Check sheet for the modelled part. Datum: model origin and axes. Units: mm. A direction names the side the tool comes from. Coordinates: 2 decimals unless noted, no trailing zeros. Loops run counter-clockwise (first coordinate to the right, second up) from the corner with the lowest first, then second, coordinate; pieces in that order, holes last. Notation, with made-up numbers: (87.5, 53) - (144.5, 53) arc R5 cw to (144.5, 58) - close; hole circle Ø5 at (38.5, -37). An arc over 180 degrees is marked (long way). Use a Markdown table: item, result. Add a question column.
1) Thickness scan on line 1 (Y direction, x = 12, z = 7.2); line 2 (X direction, y = -1.75, z = 7.5); line 3 (Z direction, x = 10.5, y = 7.25). Record the ranges inside material, lowest first.
2) Sectioned sample at B-B, the plane z = 3.75. Enter the section's corners in (x, y), then the cut area to 3 significant figures.
3) Sectioned sample at A-A, the plane z = -0.75. Enter the section's corners in (x, y).
4) Draft check along Y on faces 5 (the flat face through (12, 4, 5)), 6 (the flat face through (-12, 0, 4)), 7 (the cylindrical face through (9.5, -3.9, 7)), 8 (the flat face through (0, -8, 3)). Enter one of: pulls with the +Y half, pulls with the -Y half, needs draft (parallel to the pull), parting line crosses it, or undercut.
5) Sectioned sample at D-D, the plane y = 4. Enter the section's corners in (x, z).
6) Sectioned sample at C-C, the plane x = -12. Enter the section's corners in (y, z).
7) Go/stop test with flat-tipped pins: P1, Ø2, axis at y = 0.5, z = 7.5, coming from the -X side; P2, Ø4, axis at x = 12, y = -4, coming from the -Z side; P3, Ø4, axis at x = -10.5, y = -4.5, coming from the +Z side. Record where each tip stops, or that it passes through.
8) Tool access check on faces 1 (the flat face through (12, -4, 0)), 2 (the cylindrical face through (-1.615, 4.751, 10.986)), 3 (the flat face through (8, 2, 7)), 4 (the flat face through (-8, -4, -2)). Record the directions out of +Z, -Z, +X, -X, +Y, -Y that give a thin tool (end or side, any length) a straight path to the whole face; none if there is none.
from build123d import *

# Parameters (mm, degrees)
F0_W     = 8
F0_H     = 8
F0_R     = 2.5
F1_DEPTH = 10
F2_DEPTH = 12
F3_DEPTH = 3
F4_DEPTH = 5
F5_DEPTH = 6
F0_R_2   = 2
F6_DEPTH = 8
F7_DEPTH = 6
F8_DEPTH = 5


with BuildPart() as f1:
    # F0 (on Top) → F1 (new body)
    with BuildSketch(Plane.XY):
        with Locations((-4, 4)):
            Rectangle(F0_W, F0_H)
        with Locations((-4, 4)):
            Circle(F0_R, mode=Mode.SUBTRACT)
        with Locations((4, 4)):
            Rectangle(F0_W, F0_H)
        with Locations((4, 4)):
            Circle(F0_R, mode=Mode.SUBTRACT)
        with Locations((-4, -4)):
            Rectangle(F0_W, F0_H)
        with Locations((-4, -4)):
            Circle(F0_R, mode=Mode.SUBTRACT)
        with Locations((4, -4)):
            Rectangle(F0_W, F0_H)
        with Locations((4, -4)):
            Circle(F0_R, mode=Mode.SUBTRACT)
    extrude(amount=F1_DEPTH)

    # F0 (on Top) → F2 (join)
    with BuildSketch(Plane.XY):
        with Locations((-4, 4)):
            Circle(F0_R)
        with Locations((4, 4)):
            Circle(F0_R)
        with Locations((-4, -4)):
            Circle(F0_R)
        with Locations((4, -4)):
            Circle(F0_R)
    extrude(amount=F2_DEPTH)

    # F0 (on Top) → F3 (join)
    with BuildSketch(Plane.XY):
        with Locations((-12, 4)):
            Rectangle(F0_W, F0_H)
        with Locations((-12, 4)):
            Circle(F0_R, mode=Mode.SUBTRACT)
        with Locations((12, 4)):
            Rectangle(F0_W, F0_H)
        with Locations((12, 4)):
            Circle(F0_R, mode=Mode.SUBTRACT)
    extrude(amount=F3_DEPTH)

    # F0 (on Top) → F4 (join)
    with BuildSketch(Plane.XY):
        with Locations((-12, 4)):
            Circle(F0_R)
        with Locations((12, 4)):
            Circle(F0_R)
    extrude(amount=F4_DEPTH)

    # F0 (on Top) → F5 (join)
    with BuildSketch(Plane.XY):
        with Locations((-12, -4)):
            Rectangle(F0_W, F0_H)
        with Locations((-12, -4)):
            Circle(F0_R, mode=Mode.SUBTRACT)
        with Locations((12, -4)):
            Rectangle(F0_W, F0_H)
        with Locations((12, -4)):
            Circle(F0_R, mode=Mode.SUBTRACT)
    extrude(amount=F5_DEPTH)

    # F0 (on Top) → F6 (join)
    with BuildSketch(Plane.XY):
        with Locations((-12, -4)):
            Circle(F0_R)
        with Locations((-12, -4)):
            Circle(F0_R_2, mode=Mode.SUBTRACT)
        with Locations((12, -4)):
            Circle(F0_R)
        with Locations((12, -4)):
            Circle(F0_R_2, mode=Mode.SUBTRACT)
    extrude(amount=F6_DEPTH)

    # F0 (on Top) → F7 (join)
    with BuildSketch(Plane.XY):
        with Locations((-12, -4)):
            Circle(F0_R_2)
        with Locations((12, -4)):
            Circle(F0_R_2)
    extrude(amount=F7_DEPTH)

    # F0 (on Top) → F8 (join)
    with BuildSketch(Plane.XY):
        with Locations((-12, -4)):
            Rectangle(F0_W, F0_H)
        with Locations((-12, -4)):
            Circle(F0_R, mode=Mode.SUBTRACT)
        with Locations((12, -4)):
            Rectangle(F0_W, F0_H)
        with Locations((12, -4)):
            Circle(F0_R, mode=Mode.SUBTRACT)
    extrude(amount=-F8_DEPTH)


solid = f1.part
Solved:
| question | item | result |
|---|---|---|
| 1 | line 1 | y = -6.5 to -6, -2 to -1.5 |
| 1 | line 2 | x = -13.09 to -10.91, -8 to 8, 10.91 to 13.09 |
| 1 | line 3 | z = 0 to 3 |
| 2 | outline | (-16, -8) - (16, -8) - (16, 0) - (8, 0) - (8, 8) - (-8, 8) - (-8, 0) - (-16, 0) - close; circle Ø5 at (-12, 4); circle Ø5 at (12, 4) |
| 2 | area | 423 mm2 |
| 3 | outline | (-16, -8) - (-8, -8) - (-8, 0) - (-16, 0) - close; (8, -8) - (16, -8) - (16, 0) - (8, 0) - close; hole circle Ø5 at (-12, -4); hole circle Ø5 at (12, -4) |
| 4 | face 5 | needs draft |
| 4 | face 6 | undercut |
| 4 | face 7 | parting line crosses it |
| 4 | face 8 | pulls with the -Y half |
| 5 | outline | (-16, 0) - (16, 0) - (16, 3) - (14.5, 3) - (14.5, 5) - (9.5, 5) - (9.5, 3) - (8, 3) - (8, 10) - (6.5, 10) - (6.5, 12) - (1.5, 12) - (1.5, 10) - (-1.5, 10) - (-1.5, 12) - (-6.5, 12) - (-6.5, 10) - (-8, 10) - (-8, 3) - (-9.5, 3) - (-9.5, 5) - (-14.5, 5) - (-14.5, 3) - (-16, 3) - close |
| 6 | outline | (-8, -5) - (-6.5, -5) - (-6.5, 0) - (-1.5, 0) - (-1.5, -5) - (0, -5) - (0, 0) - (8, 0) - (8, 3) - (6.5, 3) - (6.5, 5) - (1.5, 5) - (1.5, 3) - (0, 3) - (0, 6) - (-1.5, 6) - (-1.5, 8) - (-2, 8) - (-2, 6) - (-6, 6) - (-6, 8) - (-6.5, 8) - (-6.5, 6) - (-8, 6) - close |
| 7 | P1 | stops at x = -8 |
| 7 | P2 | stops at z = 0 |
| 7 | P3 | stops at z = 8 |
| 8 | face 1 | -Z |
| 8 | face 2 | +Z |
| 8 | face 3 | +Z, +Y |
| 8 | face 4 | -Z, +Y, -Y |
